Read the model definition and answer for the solid it produces. Units are mm, in the model's axes. Give positions to 0.01 mm unless a question says otherwise; leave off trailing zeros. Order: outer loops, then holes, each group sorted by start corner. A loop starts at its lowest first (then second) coordinate and runs counter-clockwise, first axis right, second up.
Item 1: Given pin 1 Ø4 at (x, z) = (565.15, -495.3) entering from -Y, flat-ended and moving along its own axis, determine where the tip first touches the part or whether it passes through.
Item 2: A cutting plane is placed at A-A (x = 202.5). Write down the section's boundary in (y, z), plus the area to 3 significant figures.
Item 3: A cutting plane is placed at B-B (y = 2.5). State how many separate pieces and enclosed holes the cut face has, plus the area to 3 significant figures.
Item 4: Find the intervals of material crossed by line 1 along Z through (x, y) = (234.95, 4.5); line 2 along Z through (x, y) = (609.6, 3.25); line 3 along Z through (x, y) = (194, 3.75), in increasing order.
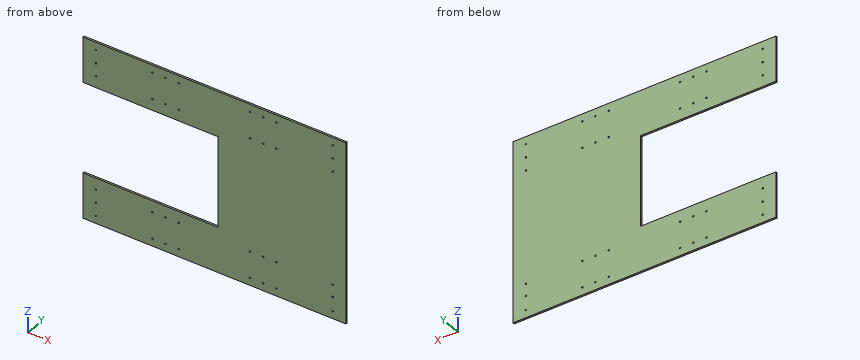
from build123d import *

# Parameters (mm, degrees)
SKETCH1_W           = 889
SKETCH1_H           = 609.6
BOSS_EXTRUDE1_DEPTH = 6.35
SKETCH2_W           = 457.2
SKETCH2_H           = 304.8
CUT_EXTRUDE1_DEPTH  = 6.35
SKETCH3_R           = 2.5527
CUT_EXTRUDE2_DEPTH  = 6.35


with BuildPart() as part:
    # Sketch1 → Boss-Extrude1 (new body)
    with BuildSketch(Plane(origin=(0, 0, 0), x_dir=(1, 0, 0), z_dir=(0, 1, 0))):
        with Locations((444.5, 304.8)):
            Rectangle(SKETCH1_W, SKETCH1_H)
    extrude(amount=BOSS_EXTRUDE1_DEPTH)

    # Sketch2 → Cut-Extrude1 (cut)
    with BuildSketch(Plane(origin=(0, 6.35, 0), x_dir=(1, 0, 0), z_dir=(0, 1, 0))):
        with Locations((228.6, 304.8)):
            Rectangle(SKETCH2_W, SKETCH2_H)
    extrude(amount=-CUT_EXTRUDE1_DEPTH, mode=Mode.SUBTRACT)

    # Sketch3 → Cut-Extrude2 (cut)
    with BuildSketch(Plane(origin=(0, 6.35, 0), x_dir=(1, 0, 0), z_dir=(0, 1, 0))):
        with Locations((44.45, 584.2)):
            Circle(SKETCH3_R)
        with Locations((44.45, 539.75)):
            Circle(SKETCH3_R)
        with Locations((44.45, 495.3)):
            Circle(SKETCH3_R)
        with Locations((44.45, 114.3)):
            Circle(SKETCH3_R)
        with Locations((44.45, 69.85)):
            Circle(SKETCH3_R)
        with Locations((44.45, 25.4)):
            Circle(SKETCH3_R)
        with Locations((234.95, 584.2)):
            Circle(SKETCH3_R)
        with Locations((279.4, 584.2)):
            Circle(SKETCH3_R)
        with Locations((323.85, 584.2)):
            Circle(SKETCH3_R)
        with Locations((234.95, 495.3)):
            Circle(SKETCH3_R)
        with Locations((279.4, 495.3)):
            Circle(SKETCH3_R)
        with Locations((323.85, 495.3)):
            Circle(SKETCH3_R)
        with Locations((234.95, 114.3)):
            Circle(SKETCH3_R)
        with Locations((279.4, 114.3)):
            Circle(SKETCH3_R)
        with Locations((323.85, 114.3)):
            Circle(SKETCH3_R)
        with Locations((234.95, 25.4)):
            Circle(SKETCH3_R)
        with Locations((279.4, 25.4)):
            Circle(SKETCH3_R)
        with Locations((323.85, 25.4)):
            Circle(SKETCH3_R)
        with Locations((565.15, 584.2)):
            Circle(SKETCH3_R)
        with Locations((565.15, 495.3)):
            Circle(SKETCH3_R)
        with Locations((609.6, 584.2)):
            Circle(SKETCH3_R)
        with Locations((609.6, 495.3)):
            Circle(SKETCH3_R)
        with Locations((654.05, 584.2)):
            Circle(SKETCH3_R)
        with Locations((654.05, 495.3)):
            Circle(SKETCH3_R)
        with Locations((565.15, 114.3)):
            Circle(SKETCH3_R)
        with Locations((609.6, 114.3)):
            Circle(SKETCH3_R)
        with Locations((654.05, 114.3)):
            Circle(SKETCH3_R)
        with Locations((565.15, 25.4)):
            Circle(SKETCH3_R)
        with Locations((609.6, 25.4)):
            Circle(SKETCH3_R)
        with Locations((654.05, 25.4)):
            Circle(SKETCH3_R)
        with Locations((844.55, 584.2)):
            Circle(SKETCH3_R)
        with Locations((844.55, 536.575)):
            Circle(SKETCH3_R)
        with Locations((844.55, 495.3)):
            Circle(SKETCH3_R)
        with Locations((844.55, 114.3)):
            Circle(SKETCH3_R)
        with Locations((844.55, 69.85)):
            Circle(SKETCH3_R)
        with Locations((844.55, 25.4)):
            Circle(SKETCH3_R)
    extrude(amount=-CUT_EXTRUDE2_DEPTH, mode=Mode.SUBTRACT)


solid = part.part
Response values:
1. pin 1: passes through
2. outline: (0, -609.6) - (6.35, -609.6) - (6.35, -457.2) - (0, -457.2) - close; (0, -152.4) - (6.35, -152.4) - (6.35, 0) - (0, 0) - close
2. area: 1,940 mm2
3. separate pieces: 1
3. enclosed holes: 36
3. area: 402,000 mm2
4. line 1: z = -609.6 to -586.75, -581.65 to -497.85, -492.75 to -457.2, -152.4 to -116.85, -111.75 to -27.95, -22.85 to 0
4. line 2: z = -609.6 to -586.75, -581.65 to -497.85, -492.75 to -116.85, -111.75 to -27.95, -22.85 to 0
4. line 3: z = -609.6 to -457.2, -152.4 to 0
